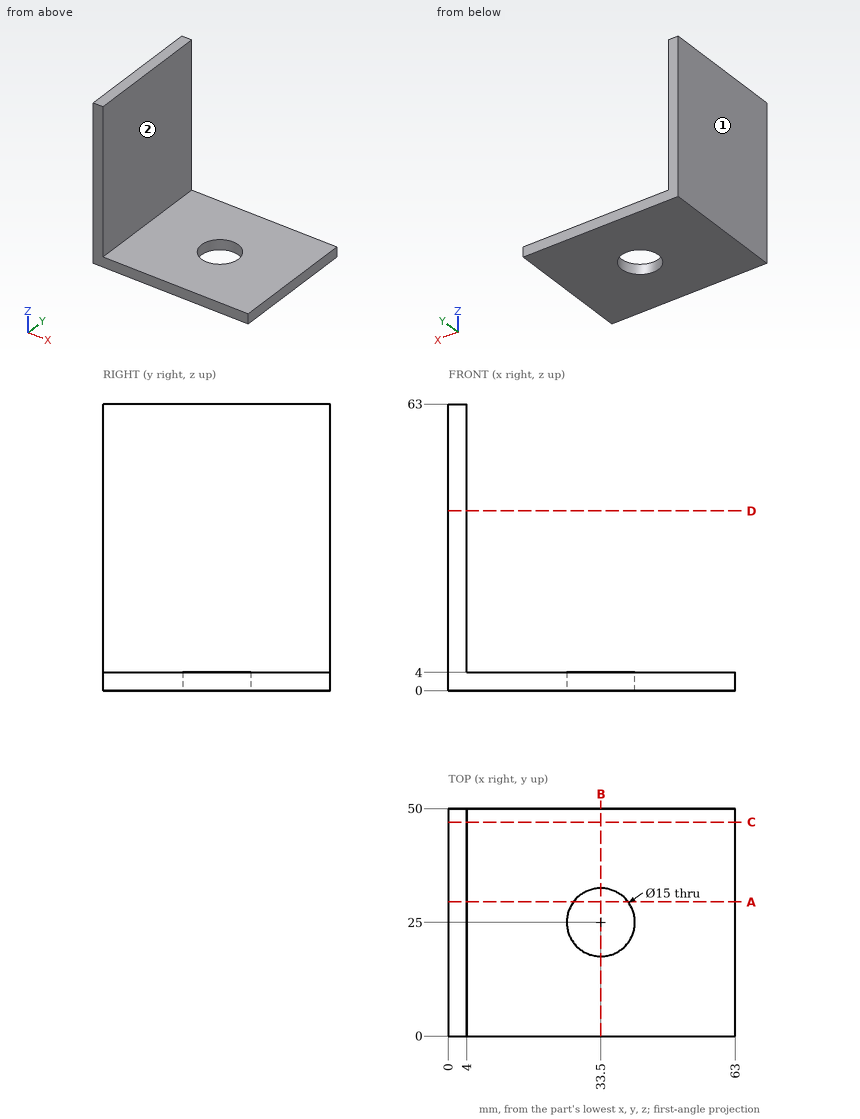
Geometry check sheet. Reference: drawing and pictorial views, mm from the part's lowest x, y, z. A direction names the side the tool comes from. Give positions to 0.01 mm unless a question says otherwise; leave off trailing zeros. Write each loop counter-clockwise with the first axis right and the second up, starting at its lowest first coordinate (ties: lowest second). Pieces come first, ordered by that corner, then holes. Notation, with made-up numbers: (30, 84) -> (76, 84) arc R24 cw to (76, 97) -> close; hole circle Ø9 at (43, 28). An arc over 180 degrees is marked (long way). One line per item, written item: value. Start each with the question number.
Item 1: Section check C-C on y = 47. Record the cut outline in (x, z).
Item 2: Section check B-B on x = 33.5. Record the cut outline in (y, z), then the cut area to 3 significant figures.
Item 3: Material ranges on probe 1 along Y at (x, z) = (33.5, 1.9); probe 2 along X at (y, z) = (39, 24.5), recorded low to high. Write a range as from..to.
Item 4: Gauge pin test, flat ends, axial feed: pin 1 (2 mm diameter, centred on x = 22, y = 28.5, fed in from -Z); pin 2 (1.5 mm diameter, centred on y = 20, z = 54, fed in from +X); pin 3 (17 mm diameter, centred on x = 33.5, y = 25, fed in from +Z). Record the tip position at first contact, or that the pin passes through.
Item 5: Tool access check on the marked faces 1 and 2. Record the directions out of +Z, -Z, +X, -X, +Y, -Y that give a thin tool (end or side, any length) a straight path to the whole face; none if there is none.
Item 6: Section check D-D on z = 39.5. Record the cut outline in (x, y), then the cut area to 3 significant figures.
Item 7: Section check A-A on y = 29.5. Record the cut outline in (x, z).
Results list:
1. outline: (0, 0) -> (63, 0) -> (63, 4) -> (4, 4) -> (4, 63) -> (0, 63) -> close
2. outline: (0, 0) -> (17.5, 0) -> (17.5, 4) -> (0, 4) -> close; (32.5, 0) -> (50, 0) -> (50, 4) -> (32.5, 4) -> close
2. area: 140 mm²
3. probe 1: 0..17.5, 32.5..50
3. probe 2: 0..4
4. pin 1: z = 0
4. pin 2: x = 4
4. pin 3: z = 4
5. face 1: +Z, -Z, -X, +Y, -Y
5. face 2: +Z, +X, +Y, -Y
6. outline: (0, 0) -> (4, 0) -> (4, 50) -> (0, 50) -> close
6. area: 200 mm²
7. outline: (0, 0) -> (27.5, 0) -> (27.5, 4) -> (4, 4) -> (4, 63) -> (0, 63) -> close; (39.5, 0) -> (63, 0) -> (63, 4) -> (39.5, 4) -> close
